```python
from build123d import *

# Parameters (mm, degrees)
BOSS_EXTRUDE1_DEPTH = 200
HOLE1_D             = 25


with BuildPart() as part:
    # Sketch1 → Boss-Extrude1 (new body)
    with BuildSketch(Plane(origin=(0, 0, 0), x_dir=(1, 0, 0), z_dir=(0, 1, 0))):
        Polygon((0, 225), (0, 250), (-150, 250), (-150, 0), (0, 0), (0, 50), (-125, 50), (-125, 225), align=None)
    extrude(amount=BOSS_EXTRUDE1_DEPTH)

    # Hole1 (through all)
    with Locations(Plane(origin=(-150, 175, -175), x_dir=(0, 0, -1), z_dir=(-1, 0, 0))):
        with Locations((0, 0), (0, 150)):
            Hole(HOLE1_D / 2)


solid = part.part
```
Here's how the part is built. I have some questions about the finished solid (model axes, mm). A direction names the side the tool comes from. Coordinates: 2 decimals unless noted, no trailing zeros. Order: outer loops, then holes, each group sorted by start corner. A loop starts at its lowest first (then second) coordinate and runs counter-clockwise, first axis right, second up. Notation, with made-up numbers: M -24.5,35 L -18.5,35 A10 ccw -18.5,51 Z; hole C -35,2.25 d6. An arc over 180 degrees is marked long. Answer as a JSON object with one key per item and string values. Group by question number.
(1) Which directions (+Z, -Z, +X, -X, +Y, -Y) give clear straight access to the entire face, cutting with the end or side of a thin tool? Please do faces 4 (the face through (-125, 99, -136)), 5 (the face through (0, 99, -25)).
(2) For pin 1 (5 mm diameter, centred on y = 127, z = -158.5, fed in from +X), with a flat end and sliding along its axis, tell me the tip position at first contact or that it passes through.
(3) I need wall thicknesses on probe 1 along Y at (x, z) = (-132, -175); probe 2 along Z at (x, y) = (-133.25, 175); probe 3 along Z at (x, y) = (-18, 110). Which ranges of each line are inside material? Lowest first, please.
(4) Suppose I cut it at D-D, the plane y = 88.5. Please give me the cut outline in (x, z), then the cut area to 3 significant figures.
(5) Suppose I cut it at C-C, the plane y = 175. Please give me the cut outline in (x, z).
(6) If we mould it in two halves opening along Z, with no side actions, what happens to faces 1 (the face through (-62, 99, -50)), 2 (the face through (-150, 99, -127)), 3 (the face through (-74, 99, -250))? For each: released by +Z, released by -Z, zero draft, split by the parting line, or undercut.
(7) Suppose I cut it at A-A, the plane x = -64.5. Please give me the cut outline in (y, z).
(8) Suppose I cut it at B-B, the plane z = -175. Please give me the cut outline in (x, y).
Values found:
{
 "1": {"face 4": "+X, +Y, -Y", "face 5": "+Z, -Z, +X, +Y, -Y"},
 "2": {"pin 1": "stops at x = -125"},
 "3": {"probe 1": "y = 0 to 12.5, 37.5 to 162.5, 187.5 to 200", "probe 2": "z = -250 to -187.5, -162.5 to 0", "probe 3": "z = -250 to -225, -50 to 0"},
 "4": {"outline": "M -150,-250 L 0,-250 L 0,-225 L -125,-225 L -125,-50 L 0,-50 L 0,0 L -150,0 Z", "area": "15,600 mm^2"},
 "5": {"outline": "M -150,-250 L 0,-250 L 0,-225 L -125,-225 L -125,-187.5 L -150,-187.5 Z; M -150,-162.5 L -125,-162.5 L -125,-50 L 0,-50 L 0,0 L -150,0 Z"},
 "6": {"face 1": "undercut", "face 2": "zero draft", "face 3": "released by -Z"},
 "7": {"outline": "M 0,-250 L 200,-250 L 200,-225 L 0,-225 Z; M 0,-50 L 200,-50 L 200,0 L 0,0 Z"},
 "8": {"outline": "M -150,0 L -125,0 L -125,12.5 L -150,12.5 Z; M -150,37.5 L -125,37.5 L -125,162.5 L -150,162.5 Z; M -150,187.5 L -125,187.5 L -125,200 L -150,200 Z"}
}
